from build123d import *

# Parameters (mm, degrees)
IZIM1_W                                      = 65
IZIM1_H                                      = 100
Y_KSEKLIK_EKSTR_ZYON1_DEPTH                  = 20
Y_KSEKLIK_EKSTR_ZYON1_DIRECTION_2_REACH      = 575.479
Y_KSEKLIK_EKSTR_ZYON1_DIRECTION_2_END_RADIUS = 1627
PAH1_SIZE                                    = 15
IZIM4_R                                      = 22.5
IZIM4_R_2                                    = 17.5
Y_KSEKLIK_EKSTR_ZYON2_DEPTH                  = 35
S_P_R1_PROFILE_R                             = 10
Y_KSEKLIK_EKSTR_ZYON3_REACH                  = 1997.162
Y_KSEKLIK_EKSTR_ZYON3_END_RADIUS             = 22.5
IZIM14_R                                     = 10


with BuildPart() as part:
    # Sketch1 → Revolve1 (revolve)
    with BuildSketch(Plane(origin=(0, 0, 0), x_dir=(0, 0, -1), z_dir=(1, 0, 0)), mode=Mode.PRIVATE) as revolve1_sk:
        with BuildLine():
            Line((-1579.017970214, -401.050482857), (-1580.413520537, -402.642399801))
            ThreePointArc((-1580.413520537, -402.642399801), (-1576.632427652, -403.522199794), (-1575, -400))
            ThreePointArc((-1575, -400), (-1612.45154966, -201.556443707), (-1625, 0))
            Line((-1625, 0), (-1627, 0))
            ThreePointArc((-1627, 0), (-1614.436105413, -201.804513177), (-1576.938461538, -400.492307692))
            ThreePointArc((-1576.938461538, -400.492307692), (-1577.702877842, -401.79718049), (-1579.017970214, -401.050482857))
        make_face()
    revolve(revolve1_sk.sketch.rotate(Axis((0, 0, 1625), (0, 0, 1)), 270), axis=Axis((0, 0, 1625), (0, 0, 1)))

    # izim1 → Y_kseklik-Ekstr_zyon1 (add)
    with BuildSketch(Plane.XY.offset(1627)):
        Rectangle(IZIM1_W, IZIM1_H)
    extrude(amount=Y_KSEKLIK_EKSTR_ZYON1_DEPTH)

    # Y_kseklik-Ekstr_zyon1 direction 2: up to this sphere (the profile starts outside it)
    y_kseklik_ekstr_zyon1_direction_2_end = Location((0, 0, 0)) * Sphere(Y_KSEKLIK_EKSTR_ZYON1_DIRECTION_2_END_RADIUS, mode=Mode.PRIVATE)
    # izim1 → Y_kseklik-Ekstr_zyon1 direction 2 (add, up to the surface)
    with BuildSketch(Plane.XY.offset(1627), mode=Mode.PRIVATE) as y_kseklik_ekstr_zyon1_direction_2_sk1:
        Rectangle(IZIM1_W, IZIM1_H)
    y_kseklik_ekstr_zyon1_direction_2_tool1 = extrude(y_kseklik_ekstr_zyon1_direction_2_sk1.sketch, amount=-Y_KSEKLIK_EKSTR_ZYON1_DIRECTION_2_REACH, mode=Mode.PRIVATE) - y_kseklik_ekstr_zyon1_direction_2_end
    add(y_kseklik_ekstr_zyon1_direction_2_tool1.solids().sort_by_distance((0, 0, 1627))[0])

    # Pah1
    pah1_edges = [part.edges().sort_by_distance(p)[0] for p in [
        (32.5, 0, 1647),
        (0, 50, 1647),
        (-32.5, 0, 1647),
        (0, -50, 1647),
    ]]
    chamfer(pah1_edges, length=PAH1_SIZE)

    # S_p_r1: sweep along a path in izim5
    with BuildLine(Plane(origin=(0, 0, 0), x_dir=(0, 0, -1), z_dir=(1, 0, 0))) as s_p_r1_path:
        Line((-1637, -627.5), (-1637, 0.081222763))
    # S_p_r1 profile (on start of the path) → S_p_r1 (sweep)
    with BuildSketch(Plane(origin=(0, -627.5, 1637), x_dir=(0, 0, 1), z_dir=(0, 1, 0))):
        Circle(S_P_R1_PROFILE_R)
    sweep(path=s_p_r1_path.line)



with BuildPart() as body_2:
    # izim4 → Y_kseklik-Ekstr_zyon2 (new, symmetric)
    with BuildSketch(Plane(origin=(0, 0, 0), x_dir=(0, 0, -1), z_dir=(1, 0, 0))):
        with Locations((-1637, -650)):
            Circle(IZIM4_R)
        with Locations((-1637, -650)):
            Circle(IZIM4_R_2, mode=Mode.SUBTRACT)
    extrude(amount=Y_KSEKLIK_EKSTR_ZYON2_DEPTH, both=True)


with BuildPart() as part_1:
    add(part.part)

    add(body_2.part)  # Y_kseklik-Ekstr_zyon3 merges body 2
    # Y_kseklik-Ekstr_zyon3: up to this cylinder (the profile starts outside it)
    y_kseklik_ekstr_zyon3_end = Plane(origin=(0, -650, 1637), z_dir=(-1, 0, 0)) * Cylinder(Y_KSEKLIK_EKSTR_ZYON3_END_RADIUS, 4040.324, mode=Mode.PRIVATE)
    # izim14 → Y_kseklik-Ekstr_zyon3 (add, up to the surface)
    with BuildSketch(Plane.XZ.offset(627.5), mode=Mode.PRIVATE) as y_kseklik_ekstr_zyon3_sk1:
        with Locations(Location((0, 1637, 0), (0, 0, 90))):
            Circle(IZIM14_R)
    y_kseklik_ekstr_zyon3_tool1 = extrude(y_kseklik_ekstr_zyon3_sk1.sketch, amount=Y_KSEKLIK_EKSTR_ZYON3_REACH, mode=Mode.PRIVATE) - y_kseklik_ekstr_zyon3_end
    add(y_kseklik_ekstr_zyon3_tool1.solids().sort_by_distance((0, -627.5, 1637))[0])
    add(y_kseklik_ekstr_zyon3_tool1.solids().sort_by_distance((0, -627.5, 1637))[1])


solid = part_1.part
For this review, take the finished solid that the model builds, in its own axes (mm). A direction names the side the tool comes from. Round coordinates to 2 decimals unless told otherwise and drop trailing zeros. Order: outer loops, then holes, each group sorted by start corner. A loop starts at its lowest first (then second) coordinate and runs counter-clockwise, first axis right, second up. Notation, with made-up numbers: (7.25, 62.25) -> (20.25, 62.25) arc R19 cw to (20.25, 81.25) -> close; hole circle Ø11 at (4, -30). An arc over 180 degrees is marked (long way). Write item = value, one per line. Start each with the question number.
1) Take a section at A-A on y = -650. State the section outline as (x, z) points.
2) Insertion check: pin 1 (1.8 mm diameter, centred on y = -14, z = 1629.5, fed in from -X); pin 2 (2 mm diameter, centred on y = -88.5, z = 1632.5, fed in from +X); pin 3 (4 mm diameter, centred on x = 247.5, y = -161, fed in from -Z). Each pin has a flat end and moves straight along its axis. Give the tip position at first contact, or say it passes through.
3) To check wall thickness, follow line 1 (Y direction, x = -19, z = 1637); line 2 (Y direction, x = 8, z = 1637); line 3 (X direction, y = -346, z = 1637). State the ranges of each line that lie inside material, in increasing order. Write a range as from..to.
4) Take a section at B-B on y = -476. State the section outline as (x, z) points, plus the area to 3 significant figures.
5) Tool access review of faces 3 (the face through (-35, -663, 1625)), 4 (the face through (0, 0, 1647)): name each direction out of +Z, -Z, +X, -X, +Y, -Y from which nothing blocks a thin tool from reaching the whole face with its end or side.
6) The part is to be moulded in two halves that separate along Y. For faces 1 (the face through (35, -663, 1625)), 2 (the face through (-0.49, -644.74, 1620.31)), say which applies: +Y half, -Y half, draft (parallel to the pull), parting line (faces both ways), or undercut.
Verdict:
q1.outline = (-35, 1614.5) -> (35, 1614.5) -> (35, 1619.5) -> (-35, 1619.5) -> close; (-35, 1654.5) -> (35, 1654.5) -> (35, 1659.5) -> (-35, 1659.5) -> close
q2.pin_1 = -32.5
q2.pin_2 = 9.37
q2.pin_3 = 1597.58
q3.line_1 = -672.5..-667.5, -632.5..-627.5, -45..45
q3.line_2 = -672.5..-667.5, -632.5..45
q3.line_3 = -10..10
q4.outline = circle Ø20 at (0, 1637)
q4.area = 314 mm2
q5.face_3 = +Z, -Z, -X, -Y
q5.face_4 = +Z, +X, -X, +Y
q6.face_1 = draft
q6.face_2 = undercut
